Part model, mm, in its own coordinate system. Face numbers are marked on the shaded views. A direction names the side the tool comes from. Round coordinates to 2 decimals unless told otherwise and drop trailing zeros. Order: outer loops, then holes, each group sorted by start corner. A loop starts at its lowest first (then second) coordinate and runs counter-clockwise, first axis right, second up. Notation, with made-up numbers: (28.5, -10) - (33.5, -10) arc R26 cw to (33.5, 26) - close; hole circle Ø2 at (36, 15). An arc over 180 degrees is marked (long way). Answer as a JSON object with one key per item and string values.
```python
from build123d import *

# Parameters (mm, degrees)
SKETCH_1_W          = 94
SKETCH_1_H          = 34
EXTRUDE_1_DEPTH     = 2.5
SKETCH_2_W          = 94
SKETCH_2_H          = 34
SKETCH_2_W_2        = 44
SKETCH_2_H_2        = 30
EXTRUDE_2_DEPTH     = 25
CUT_EXTRUDE_1_DEPTH = 104.038827633
SKETCH_7_R          = 5
EXTRUDE_4_DEPTH     = 34
SKETCH_8_R          = 1.5
CUT_EXTRUDE_2_DEPTH = 104.038827633


with BuildPart() as part:
    # 草图1 → 凸台-拉伸1 (new body)
    with BuildSketch(Plane(origin=(0, 0, 0), x_dir=(1, 0, 0), z_dir=(0, 1, 0))):
        with Locations((47, 17)):
            Rectangle(SKETCH_1_W, SKETCH_1_H)
    extrude(amount=EXTRUDE_1_DEPTH)

    # 草图2 → 凸台-拉伸2 (add)
    with BuildSketch(Plane(origin=(0, 0, 0), x_dir=(-1, 0, 0), z_dir=(0, -1, 0))):
        with Locations((-47, 17)):
            Rectangle(SKETCH_2_W, SKETCH_2_H)
        with Locations((-24, 17)):
            Rectangle(SKETCH_2_W_2, SKETCH_2_H_2, mode=Mode.SUBTRACT)
        with Locations((-70, 17)):
            Rectangle(SKETCH_2_W_2, SKETCH_2_H_2, mode=Mode.SUBTRACT)
    extrude(amount=EXTRUDE_2_DEPTH)

    # 草图6 → 切除-拉伸1 (cut, through all)
    with BuildSketch(Plane(origin=(0, 0, -34), x_dir=(-1, 0, 0), z_dir=(0, 0, -1))):
        Polygon((0, -25), (0, 1), (-46, -25), align=None)
        Polygon((-94, -25), (-94, 1), (-48, -25), align=None)
    extrude(amount=-CUT_EXTRUDE_1_DEPTH, mode=Mode.SUBTRACT)

    # 草图7 → 凸台-拉伸4 (add)
    with BuildSketch(Plane(origin=(0, 0, -34), x_dir=(-1, 0, 0), z_dir=(0, 0, -1))):
        with Locations((-47, -2.5)):
            Circle(SKETCH_7_R)
    extrude(amount=-EXTRUDE_4_DEPTH)

    # 草图8 → 切除-拉伸2 (cut, through all)
    with BuildSketch(Plane(origin=(0, 0, -34), x_dir=(-1, 0, 0), z_dir=(0, 0, -1))):
        with Locations((-47, -2.5)):
            Circle(SKETCH_8_R)
    extrude(amount=-CUT_EXTRUDE_2_DEPTH, mode=Mode.SUBTRACT)


solid = part.part
```
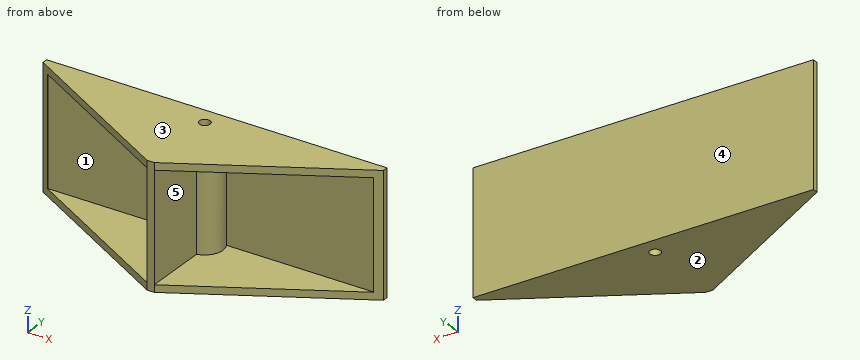
Item 1: Cut at A-A (x = 47). Write the cut outline in (y, z).
Taken from the geometry:
{"outline": "(-25, -34) - (-4, -34) - (-4, 0) - (-25, 0) - close; (-1, -34) - (2.5, -34) - (2.5, 0) - (-1, 0) - close"}
Item 2: Drop flat-ended pins along their axis: P1, Ø3, axis at y = -1.5, z = -27.5, coming from the -X side; P2, Ø5.5, axis at y = -17.5, z = -22.5, coming from the +X side; P3, Ø9, axis at y = -16, z = -20.5, coming from the -X side. Give the stop position or say it passes through.
Taken from the geometry:
{"P1": "x = 1.77", "P2": "x = 48", "P3": "x = 46"}
Item 3: Probe L1, parallel to Y at x = 47, z = -21; L2, parallel to Z at x = 50, y = -11.75; L3, parallel to X at y = -11.75, z = -26. List the from-to ranges inside material, lowest first. Write a range as from..to.
Taken from the geometry:
{"L1": "-25..-4, -1..2.5", "L2": "-34..-32, -2..0", "L3": "46..48"}
Item 4: Tool access for the marked faces 4 and 5: list every direction of +Z, -Z, +X, -X, +Y, -Y with a clear straight run to the whole face (end or side of a thin tool).
Taken from the geometry:
{"face 4": "+Z, -Z, +X, -X, +Y", "face 5": "+X, -Y"}
Item 5: Two-plate mould, pull along Z, no slides. Class the marked faces 1, 2 and 3: pulls with the +Z half, pulls with the -Z half, needs draft (parallel to the pull), parting line crosses it, or undercut.
Taken from the geometry:
{"face 1": "undercut", "face 2": "pulls with the -Z half", "face 3": "pulls with the +Z half"}
Item 6: Cut at D-D (x = 60). Write the cut outline in (y, z).
Taken from the geometry:
{"outline": "(-18.22, -34) - (2.5, -34) - (2.5, 0) - (-18.22, 0) - (-18.22, -2) - (0, -2) - (0, -32) - (-18.22, -32) - close"}
Item 7: Cut at B-B (z = -13). Write the cut outline in (x, y), plus the area to 3 significant figures.
Taken from the geometry:
{"outline": "(0, 1) - (2, -0.13) - (2, 0) - (42.67, 0) arc R5 ccw to (46, -7.4) - (46, -25) - (48, -25) - (48, -7.4) arc R5 ccw to (51.33, 0) - (92, 0) - (92, -0.13) - (94, 1) - (94, 2.5) - (0, 2.5) - close; hole circle Ø3 at (47, -2.5)", "area": "324 mm2"}
Item 8: Cut at C-C (y = -2.5). Write the cut outline in (x, z), plus the area to 3 significant figures.
Taken from the geometry:
{"outline": "(6.19, -34) - (45.5, -34) - (45.5, 0) - (6.19, 0) - (6.19, -2) - (42, -2) - (42, -32) - (6.19, -32) - close; (48.5, -34) - (87.81, -34) - (87.81, -32) - (52, -32) - (52, -2) - (87.81, -2) - (87.81, 0) - (48.5, 0) - close", "area": "524 mm2"}
